Read the model definition and answer for the solid it produces. Units are mm, in the model's axes. Face numbers are marked on the shaded views. A direction names the side the tool comes from. Coordinates: 2 decimals unless noted, no trailing zeros. Order: outer loops, then holes, each group sorted by start corner. A loop starts at its lowest first (then second) coordinate and runs counter-clockwise, first axis right, second up. Notation, with made-up numbers: M 10,14.25 L 33,14.25 A28 cw 33,38.25 Z; hole C 7,3.5 d7. An arc over 180 degrees is marked long. One line per question, with ' | ' between items. Start each with the question number.
1) Find section B-B, the plane x = 51.5. Write down the section's boundary in (y, z), plus the area to 3 significant figures.
2) Find section D-D, the plane y = 41. Write down the section's boundary in (x, z), plus the area to 3 significant figures.
3) Given P1, Ø0.6, axis at x = -36, y = 30, coming from the +Z side; P2, Ø6, axis at y = 22, z = 1, coming from the +X side; P3, Ø3, axis at y = 15.5, z = 2, coming from the -X side; P4, Ø1, axis at x = 15, z = 1.5, coming from the -Y side, each flat-ended and moving along its own axis, determine where each tip first touches the part or whether it passes through.
4) Find section C-C, the plane y = 25. Write down the section's boundary in (x, z), plus the area to 3 significant figures.
5) Find section A-A, the plane z = -1.75. Write down the section's boundary in (x, y), plus the area to 3 significant figures.
6) Consider probe 1 along X at (y, z) = (2, 4.5); probe 2 along Y at (x, z) = (12, 7.75); probe 3 along Y at (x, z) = (-49.5, 3.25). Determine where each line is inside the solid, lowest interval first.
7) A tool of negligible diameter and unlimited length cuts with its end or side. For the marked faces 1, 2, 3, 4 and 5, from which of +Z, -Z, +X, -X, +Y, -Y can it reach the whole face along a straight path? Write none if from no direction.
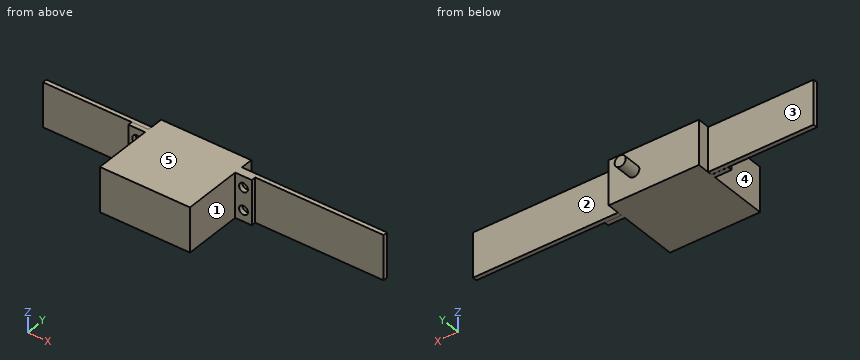
from build123d import *

# Parameters (mm, degrees)
SKETCH1_W                = 40.5
SKETCH1_H                = 20
BOSS_EXTRUDE1_DEPTH      = 36.1
SKETCH2_R                = 2.5
BOSS_EXTRUDE2_DEPTH      = 8
BOSS_EXTRUDE3_DEPTH      = 7.5
BOSS_EXTRUDE3_DEPTH_BACK = 48
SKETCH3_W                = 20
SKETCH3_H                = 2
SKETCH4_R                = 2
CUT_EXTRUDE1_DEPTH       = 7.5
SKETCH5_W                = 47.383386501
SKETCH5_H                = 19.900048315
SKETCH5_W_2              = 65.196690676
SKETCH5_H_2              = 19.999647671
BOSS_EXTRUDE4_DEPTH      = 2


with BuildPart() as part:
    # Sketch1 → Boss-Extrude1 (new body)
    with BuildSketch(Plane(origin=(0, 0, 0), x_dir=(1, 0, 0), z_dir=(0, 1, 0))):
        with Locations((3.506737992, 0.753901676)):
            Rectangle(SKETCH1_W, SKETCH1_H)
    extrude(amount=BOSS_EXTRUDE1_DEPTH)

    # Sketch2 → Boss-Extrude2 (add)
    with BuildSketch(Plane(origin=(0, 36.1, 0), x_dir=(1, 0, 0), z_dir=(0, 1, 0))):
        with Locations(Location((12.506737992, 0.753901676, 0), (0, 0, 270))):
            Circle(SKETCH2_R)
    extrude(amount=BOSS_EXTRUDE2_DEPTH)

    # Sketch3 → Boss-Extrude3 (add, two sides: drawn at the far end of the back side and taken through both)
    with BuildSketch(Plane.ZY.offset(16.743262008).offset(-BOSS_EXTRUDE3_DEPTH_BACK)):
        with Locations((-0.753901676, 27.6)):
            Rectangle(SKETCH3_W, SKETCH3_H)
    extrude(amount=BOSS_EXTRUDE3_DEPTH + BOSS_EXTRUDE3_DEPTH_BACK)

    # Sketch4 → Cut-Extrude1 (cut)
    with BuildSketch(Plane(origin=(0, 28.6, 0), x_dir=(1, 0, 0), z_dir=(0, 1, 0))):
        with Locations(Location((-20.493262008, 5.753901676, 0), (0, 0, 270))):
            Circle(SKETCH4_R)
        with Locations(Location((27.506737992, 5.753901676, 0), (0, 0, 270))):
            Circle(SKETCH4_R)
        with Locations(Location((-20.493262008, -4.246098324, 0), (0, 0, 270))):
            Circle(SKETCH4_R)
        with Locations(Location((27.506737992, -4.246098324, 0), (0, 0, 270))):
            Circle(SKETCH4_R)
    extrude(amount=-CUT_EXTRUDE1_DEPTH, mode=Mode.SUBTRACT)

    # Sketch5 → Boss-Extrude4 (add)
    with BuildSketch(Plane(origin=(0, 28.6, 0), x_dir=(1, 0, 0), z_dir=(0, 1, 0))):
        with Locations((-40.434955259, 0.760670561)):
            Rectangle(SKETCH5_W, SKETCH5_H)
        with Locations((56.35508333, 0.753725511)):
            Rectangle(SKETCH5_W_2, SKETCH5_H_2)
    extrude(amount=BOSS_EXTRUDE4_DEPTH)


solid = part.part
Report:
1) outline: M 28.6,-10.75 L 30.6,-10.75 L 30.6,9.25 L 28.6,9.25 Z | area: 40.0 mm^2
2) outline: C 12.51,-0.75 d5 | area: 19.6 mm^2
3) P1: stops at z = 9.19 | P2: stops at x = 23.76 | P3: stops at x = -16.74 | P4: stops at y = 0
4) outline: M -16.74,-10.75 L 23.76,-10.75 L 23.76,9.25 L -16.74,9.25 Z | area: 810 mm^2
5) outline: M -64.13,28.6 L -24.24,28.6 L -24.24,26.6 L -16.74,26.6 L -16.74,0 L 23.76,0 L 23.76,26.6 L 31.26,26.6 L 31.26,28.6 L 88.95,28.6 L 88.95,30.6 L 23.76,30.6 L 23.76,36.1 L 14.8,36.1 L 14.8,44.1 L 10.21,44.1 L 10.21,36.1 L -16.74,36.1 L -16.74,30.6 L -64.13,30.6 Z | area: 1,750 mm^2
6) probe 1: x = -16.74 to 23.76 | probe 2: y = 0 to 36.1 | probe 3: y = 28.6 to 30.6
7) face 1: +Z, -Z, +X, -Y | face 2: +Z, -Z, +X, +Y | face 3: +Z, -Z, -X, +Y | face 4: +Z, -Z, -X, -Y | face 5: +Z, +X, -X, +Y, -Y
